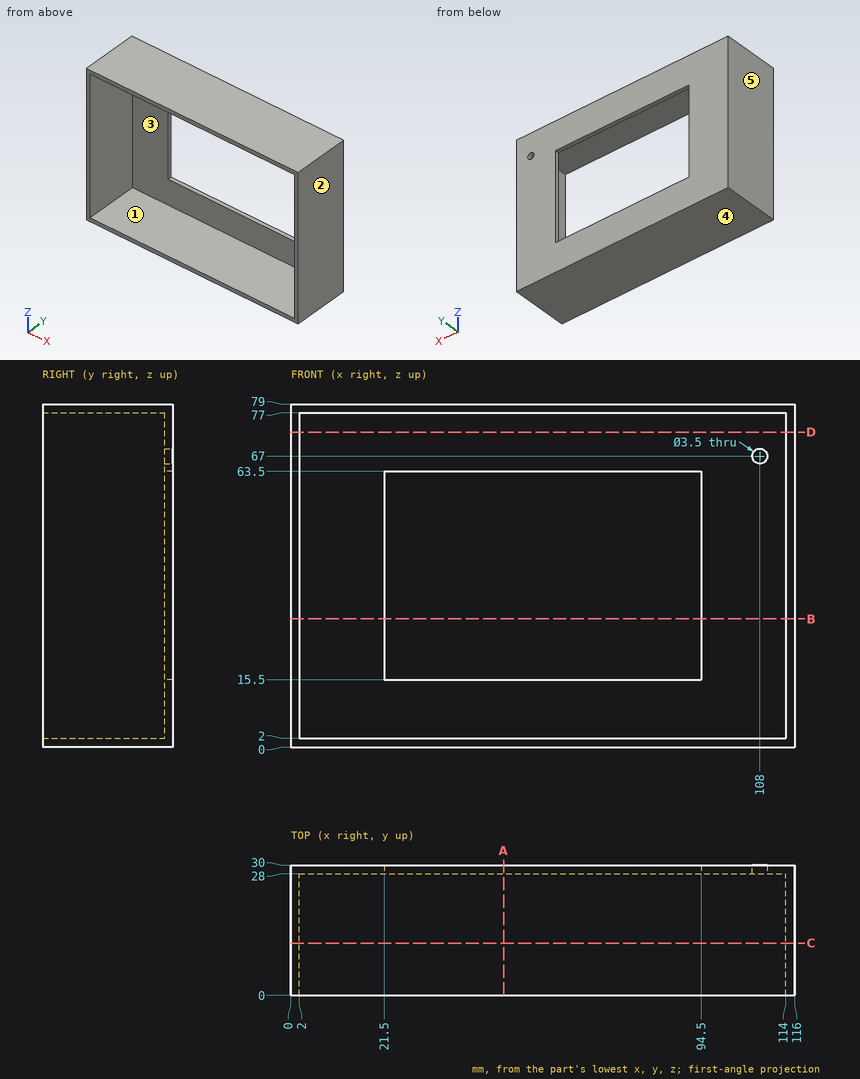
Answer from the drawing. Dimensions are ordinates in mm from the lowest x, y and z of the part. A direction names the side the tool comes from. Coordinates: 2 decimals unless noted, no trailing zeros. Loops run counter-clockwise (first coordinate to the right, second up) from the corner with the lowest first, then second, coordinate; pieces in that order, holes last.
1) Section D-D (z = 72.5) is taken. Give the vertices of the cut face in (x, y).
Results:
outline: (0, 0) - (2, 0) - (2, 28) - (114, 28) - (114, 0) - (116, 0) - (116, 30) - (0, 30) - close
2) For the marked faces 1 and 2, determine the directions among +Z, -Z, +X, -X, +Y, -Y from which every point of the face is accessible in a straight line to the end or side of a thin tool.
Results:
face 1: -Y
face 2: +Z, -Z, +X, +Y, -Y
3) Consider probe 1 along X at (y, z) = (28.5, 67); probe 2 along Z at (x, y) = (55, 1.75); probe 3 along Z at (x, y) = (108, 29.2). Determine where each line is inside the solid, lowest interval first.
Results:
probe 1: x = 0 to 106.25, 109.75 to 116
probe 2: z = 0 to 2, 77 to 79
probe 3: z = 0 to 65.25, 68.75 to 79
4) A flat-ended cylindrical pin translates along its axis: pin 1 (3 mm diameter, centred on x = 108, z = 67, fed in from +Y). Find the tip coordinate at first contact, or state that the pin passes through.
Results:
pin 1: passes through
5) For a pull along X with two mould halves and no side action, classify the marked faces 3, 4 and 5 as +X half, -X half, draft (parallel to the pull), parting line (faces both ways), or undercut.
Results:
face 3: undercut
face 4: draft
face 5: -X half
6) Section B-B (z = 29.5) is taken. Give the vertices of the cut face in (x, y).
Results:
outline: (0, 0) - (2, 0) - (2, 28) - (21.5, 28) - (21.5, 30) - (0, 30) - close; (94.5, 28) - (114, 28) - (114, 0) - (116, 0) - (116, 30) - (94.5, 30) - close
7) Section A-A (x = 49) is taken. Give the vertices of the cut face in (y, z), plus the area to 3 significant figures.
Results:
outline: (0, 0) - (30, 0) - (30, 15.5) - (28, 15.5) - (28, 2) - (0, 2) - close; (0, 77) - (28, 77) - (28, 63.5) - (30, 63.5) - (30, 79) - (0, 79) - close
area: 174 mm2
8) Section C-C (y = 12) is taken. Give the vertices of the cut face in (x, z), plus the area to 3 significant figures.
Results:
outline: (0, 0) - (116, 0) - (116, 79) - (0, 79) - close; hole (2, 2) - (114, 2) - (114, 77) - (2, 77) - close
area: 764 mm2
